```python
from build123d import *

# Parameters (mm, degrees)
F0_R     = 6
F1_DEPTH = 2
F2_R     = 2.45
F3_DEPTH = 8
F4_SIZE  = 0.3
F5_SIZE  = 0.2


with BuildPart() as f1:
    # F0 (on Top) → F1 (new body)
    with BuildSketch(Plane.XY):
        Circle(F0_R)
    extrude(amount=F1_DEPTH)

    # F2 (on face) → F3 (join)
    with BuildSketch(Plane.XY.offset(2)):
        Circle(F2_R)
    extrude(amount=F3_DEPTH)

    # F4
    f4_edges = [f1.edges().sort_by_distance(p)[0] for p in [
        (-2.45, 0, 10),
    ]]
    chamfer(f4_edges, length=F4_SIZE)

    # F5
    f5_edges = [f1.edges().sort_by_distance(p)[0] for p in [
        (-6, 0, 2),
        (-6, 0, 0),
    ]]
    chamfer(f5_edges, length=F5_SIZE)


solid = f1.part
```
The model under review builds one solid part; all positions refer to its coordinate system, in mm. A direction names the side the tool comes from. Round coordinates to 2 decimals unless told otherwise and drop trailing zeros. Loops run counter-clockwise (first coordinate to the right, second up) from the corner with the lowest first, then second, coordinate; pieces in that order, holes last. Notation, with made-up numbers: (84.25, -6.5) -> (103.25, -6.5) arc R21 cw to (103.25, 8.5) -> close; hole circle Ø1 at (-8, 28.5). An arc over 180 degrees is marked (long way). Answer in a Markdown table with one row per item.
1) Wall thickness on line 1 along Z through (x, y) = (0.5, 4.5); line 2 along Y through (x, z) = (0, 3); line 3 along Y through (x, z) = (1.25, 1.5): over which ranges is each line inside the solid? List them lowest first.
Taken from the geometry:
| item | result |
|---|---|
| line 1 | z = 0 to 2 |
| line 2 | y = -2.45 to 2.45 |
| line 3 | y = -5.87 to 5.87 |
2) Consider section C-C, the plane z = 6. Write out the cut boundary in (x, y).
Taken from the geometry:
| item | result |
|---|---|
| outline | circle Ø4.9 at (0, 0) |
3) Tool access review of faces 1 (the flat face through (0, 0, 10)), 2 (the flat face through (2.5, -1.2, 2)): name each direction out of +Z, -Z, +X, -X, +Y, -Y from which nothing blocks a thin tool from reaching the whole face with its end or side.
Taken from the geometry:
| item | result |
|---|---|
| face 1 | +Z, +X, -X, +Y, -Y |
| face 2 | +Z |
4) Consider section A-A, the plane x = 0. Write out the cut boundary in (y, z).
Taken from the geometry:
| item | result |
|---|---|
| outline | (-6, 0.2) -> (-5.8, 0) -> (5.8, 0) -> (6, 0.2) -> (6, 1.8) -> (5.8, 2) -> (2.45, 2) -> (2.45, 9.7) -> (2.15, 10) -> (-2.15, 10) -> (-2.45, 9.7) -> (-2.45, 2) -> (-5.8, 2) -> (-6, 1.8) -> close |
5) For pin 1 Ø3 at (x, z) = (-4, 4) entering from +Y; pin 2 Ø2 at (y, z) = (-3, 8.5) entering from -X; pin 3 Ø1.5 at (x, z) = (-1.5, 3.5) entering from -Y, all flat-tipped, find the tip position at first contact; note any pin that passes through.
Taken from the geometry:
| item | result |
|---|---|
| pin 1 | passes through |
| pin 2 | stops at x = -1.42 |
| pin 3 | stops at y = -2.33 |
6) Consider section D-D, the plane z = 0.5. Write out the cut boundary in (x, y).
Taken from the geometry:
| item | result |
|---|---|
| outline | circle Ø12 at (0, 0) |
